Autodesk Inventor part; units mm, degrees
ref_plane "YZ Plane" through (0, 0, 0) normal (1, 0, 0) x (0, 1, 0)
ref_plane "XZ Plane" through (0, 0, 0) normal (0, 1, 0) x (-1, 0, 0)
ref_plane "XY Plane" through (0, 0, 0) normal (0, 0, 1) x (1, 0, 0)
sketch "Sketch1" plane through (0, 0, 0) normal (0, 0, 1) x (1, 0, 0)
  line L0 (0, -139.3108) -> (63.5, -139.3108)
  line L1 (63.5, -139.3108) -> (63.5, 101.9892)
  line L2 (63.5, 101.9892) -> (0, 101.9892)
  line L3 (0, 101.9892) -> (0, -139.3108)
  point P0 (0, 0)
  dimension "d0" = 63.5
  dimension "d1" = 241.3
extrude "Extrusion1" add sketch "Sketch1" along normal blind 12.7
hole "Hole15" at (8.128, -134.3578, 12.7) direction (0, 0, -1) diameter 5.08 end through all
hole "Hole16" at (55.372, -134.3578, 12.7) direction (0, 0, -1) diameter 5.08 end through all
hole "Hole17" at (8.128, -87.1138, 12.7) direction (0, 0, -1) diameter 5.08 end through all
hole "Hole18" at (55.372, -87.1138, 12.7) direction (0, 0, -1) diameter 5.08 end through all
hole "Hole19" at (31.75, -63.1108, 12.7) direction (0, 0, -1) diameter 9.525 end through all
hole "Hole20" at (31.75, -110.7358, 12.7) direction (0, 0, -1) diameter 19.05 end through all
sketch "Font" plane through (0, 0, 12.7) normal (0, 0, 1) x (1, 0, 0)
  circle A0 centre (31.75, -110.7358) radius 9.525
  circle A1 centre (31.75, -63.1108) radius 4.7625
  circle A2 centre (55.372, -87.1138) radius 2.54
  circle A3 centre (8.128, -87.1138) radius 2.54
  circle A4 centre (55.372, -134.3578) radius 2.54
  circle A5 centre (8.128, -134.3578) radius 2.54
  line L0 (0, -139.3108) -> (0, 101.9892)
  line L1 (63.5, -139.3108) -> (0, -139.3108)
  line L2 (63.5, 101.9892) -> (63.5, -139.3108)
  line L3 (0, 101.9892) -> (63.5, 101.9892)
  point P0 (0, 0)
  dimension "d220" = 241.3
  dimension "d221" = 5.08
  dimension "d222" = 9.525
  dimension "d223" = 19.05
  dimension "d224" = 8.128
  dimension "d225" = 4.953
  dimension "d226" = 28.575
  dimension "d227" = 76.2
  dimension "d228" = 8.128
  dimension "d229" = 4.953
  dimension "d230" = 52.197
  dimension "d231" = 52.197
  dimension "d238" = 31.75
sketch "bottom" plane through (0, -139.3108, 0) normal (0, -1, 0) x (1, 0, 0)
  line L0 (63.5, 12.7) -> (0, 12.7)
  line L1 (0, 0) -> (0, 12.7)
  line L2 (0, 0) -> (63.5, 0)
  line L3 (63.5, 0) -> (63.5, 12.7)
  point P0 (47.752, 6.35)
  point P1 (15.748, 6.35)
  dimension "d233" = 12.7
sketch "Right" plane through (63.5, -139.3108, 0) normal (1, 0, 0) x (0, 0, -1)
  line L0 (-12.7, 241.3) -> (-12.7, 0)
  line L1 (0, 0) -> (-12.7, 0)
  line L2 (0, 0) -> (0, 241.3)
  line L3 (0, 241.3) -> (-12.7, 241.3)
  point P0 (0, 139.3108)
hole "Hole25" at (63.5, -126.6108, 6.35) direction (-1, 0, 0) diameter 4.826 depth 19.05 tip angle 118
hole "Hole26" at (63.5, -101.2108, 6.35) direction (-1, 0, 0) diameter 4.826 depth 19.05 tip angle 118
sketch "Sketch6" plane through (63.5, -139.3108, 0) normal (1, 0, 0) x (0, 0, -1)
  circle A0 centre (-6.35, 38.1) radius 2.413
  circle A1 centre (-6.35, 12.7) radius 2.413
  line L0 (-12.7, 241.3) -> (-12.7, 0)
  line L1 (0, 0) -> (-12.7, 0)
  line L2 (0, 0) -> (0, 241.3)
  line L3 (0, 241.3) -> (-12.7, 241.3)
  point P0 (0, 139.3108)
  dimension "d257" = 4.826
  dimension "d260" = 38.1
  dimension "d261" = 12.7
properties part number "xtower1"
Geometry: final body of the model. Coordinates: model frame, mm. A direction names the side the tool comes from. Round coordinates to 2 decimals unless told otherwise and drop trailing zeros. Write each loop counter-clockwise with the first axis right and the second up, starting at its lowest first coordinate (ties: lowest second). Pieces come first, ordered by that corner, then holes. Notation, with made-up numbers: M 30,88 L 49,88 A19 cw 49,92 Z; hole C -7.75,12 d4. An arc over 180 degrees is marked long. Answer in a Markdown table with one row per item. Add a question column.
(1) Contact query for flat-ended pins moving along their axis: pin 1 (5.5 mm diameter, centred on x = 31.75, y = -63.11, fed in from +Z); pin 2 (4 mm diameter, centred on y = -126.61, z = 6.35, fed in from +X). Output: stop coordinate, or through.
(2) Ray query, L1, parallel to Y at x = 52.75, z = 6.35; L2, parallel to Y at x = 55, z = 6.35; L3, parallel to Y at x = 29, z = 1.5. Return the intervals inside material, ascending.
(3) Cut plane A-A, the plane x = 31.75. Return the cut outline in (y, z).
(4) Draft query along X for faces 1 (the face through (53.8, -129, 6.7)), 2 (the face through (8.02, -131.82, 6.26)), 3 (the face through (0, -17, 6)). Return one class per face: pulls with the +X half, pulls with the -X half, needs draft (parallel to the pull), parting line crosses it, or undercut.
(5) Reachability of faces 4 (the face through (57.85, -86.56, 6.26)), 5 (the face through (53.842, -98.855, 6.873)) from +Z, -Z, +X, -X, +Y, -Y: full face, straight path, thin tool, end or side. Return the list, or none.
(6) Cut plane B-B, the plane y = -117. Return the cut outline in (x, z).
Established:
| question | item | result |
|---|---|---|
| 1 | pin 1 | through |
| 1 | pin 2 | x = 44.2 |
| 2 | L1 | -139.31 to -129.02, -124.2 to -103.62, -98.8 to 101.99 |
| 2 | L2 | -139.31 to -136.87, -131.85 to -129.02, -124.2 to -103.62, -98.8 to -89.63, -84.6 to 101.99 |
| 2 | L3 | -139.31 to -119.86, -101.62 to -67, -59.22 to 101.99 |
| 3 | outline | M -139.31,0 L -120.26,0 L -120.26,12.7 L -139.31,12.7 Z; M -101.21,0 L -67.87,0 L -67.87,12.7 L -101.21,12.7 Z; M -58.35,0 L 101.99,0 L 101.99,12.7 L -58.35,12.7 Z |
| 4 | face 1 | needs draft |
| 4 | face 2 | undercut |
| 4 | face 3 | pulls with the -X half |
| 5 | face 4 | +Z, -Z |
| 5 | face 5 | +X |
| 6 | outline | M 0,0 L 24.57,0 L 24.57,12.7 L 0,12.7 Z; M 38.93,0 L 63.5,0 L 63.5,12.7 L 38.93,12.7 Z |
